Build history of the part. All positions in model axes, mm. A direction names the side the tool comes from. Round coordinates to 2 decimals unless told otherwise and drop trailing zeros. Order: outer loops, then holes, each group sorted by start corner. A loop starts at its lowest first (then second) coordinate and runs counter-clockwise, first axis right, second up. Notation, with made-up numbers: M -16.5,88.25 L 17.5,88.25 A6 ccw 17.5,94.25 Z; hole C 24.5,-25 d2. An arc over 180 degrees is marked long. One line per item, written item: value. Start each with the question number.
Item 1: Band-saw the part on D-D, the plane x = 37. Write the cut outline in (y, z).
Item 2: Pin check, flat tips, straight feed: pin 1 (0.6 mm diameter, centred on x = 26, y = 1, fed in from +Z); pin 2 (3.5 mm diameter, centred on x = 45.48, z = -41.7, fed in from +Y). Stop position of each tip, or through.
Item 3: Tool access for faces 5 (the flat face through (10, 1, -39.701)), 6 (the flat face through (37, 2, -37)), 7 (the flat face through (23, 1, -36.692)): list every direction of +Z, -Z, +X, -X, +Y, -Y with a clear straight run to the whole face (end or side of a thin tool).
Item 4: Probe L1, parallel to Z at x = 11, y = 1.3; L2, parallel to X at y = 0.8, z = -6; L3, parallel to Z at x = 45.48, y = 1.65. List the from-to ranges inside material, lowest first.
Item 5: Two-plate mould, pull along Z, no slides. Class faces 1 (the flat face through (0, 1, -43)), 2 (the flat face through (41.967, 0.986, 18.527)), 3 (the flat face through (10, 1, -43.701)), 4 (the flat face through (4.55, 1, -42)): +Z half, -Z half, draft (parallel to the pull), parting line (faces both ways), or undercut.
Item 6: Band-saw the part on A-A, the plane x = 8.5. Write the cut outline in (y, z).
Item 7: Band-saw the part on C-C, the plane z = -21. Write the cut outline in (x, y).
Item 8: Band-saw the part on B-B, the plane y = 0.6. Write the cut outline in (x, z), then the cut area to 3 significant figures.
```python
from build123d import *

# Parameters (mm, degrees)
SKETCH1_R           = 2
BOSS_EXTRUDE2_DEPTH = 2
CUT_EXTRUDE2_DEPTH  = 9
CUT_EXTRUDE3_DEPTH  = 9


with BuildPart() as part:
    # Sketch1 → Boss-Extrude2 (new body)
    with BuildSketch(Plane(origin=(0, 0, 0), x_dir=(1, 0, 0), z_dir=(0, 1, 0))):
        with BuildLine():
            Line((0, 48.412862342), (0, 37.692030173))
            ThreePointArc((0, 37.692030173), (0.292893219, 36.984923392), (1, 36.692030173))
            Line((1, 36.692030173), (31.48, 36.692030173))
            Line((31.48, 36.692030173), (43.036527631, 36.692030173))
            Line((43.036527631, 36.692030173), (43.036527631, -13.307969827))
            Line((43.036527631, -13.307969827), (38.310297741, -17.310739702))
            Line((38.310297741, -17.310739702), (34.253582629, -17.310739702))
            Line((34.253582629, -17.310739702), (36, -19.267392345))
            Line((36, -19.267392345), (30.071702425, -24.288225334))
            Line((30.071702425, -24.288225334), (54.200832168, -12.602889922))
            Line((54.200832168, -12.602889922), (54.200832168, 10.267562985))
            Line((54.200832168, 10.267562985), (54.200832168, 49.412862342))
            Line((54.200832168, 49.412862342), (41.48, 49.412862342))
            Line((41.48, 49.412862342), (1, 49.412862342))
            ThreePointArc((1, 49.412862342), (0.292893219, 49.119969123), (0, 48.412862342))
        make_face()
        with Locations((45.48, 41.700609081)):
            Circle(SKETCH1_R, mode=Mode.SUBTRACT)
        with BuildLine():
            Line((15, 43.700609081), (4.549516448, 43.700609081))
            Line((4.549516448, 43.700609081), (4.549516448, 39.700609081))
            Line((4.549516448, 39.700609081), (15, 39.700609081))
            ThreePointArc((15, 39.700609081), (17, 41.700609081), (15, 43.700609081))
        make_face(mode=Mode.SUBTRACT)
    extrude(amount=BOSS_EXTRUDE2_DEPTH)

    # Sketch6 → Cut-Extrude2 (cut)
    with BuildSketch(Plane(origin=(0, 2, 0), x_dir=(1, 0, 0), z_dir=(0, 1, 0))):
        Polygon((36, -19.267392345), (38.310297741, -17.310739702), (34.253582629, -17.310739702), align=None)
    extrude(amount=-CUT_EXTRUDE2_DEPTH, mode=Mode.SUBTRACT)

    # Sketch8 → Cut-Extrude3 (cut)
    with BuildSketch(Plane(origin=(0, 2, 0), x_dir=(1, 0, 0), z_dir=(0, 1, 0))):
        Polygon((43.036527631, 36.692030173), (45.036527631, 36.692030173), (45.036527631, -11.115496155), (45.036527631, -11.614116599), (43.036527631, -13.307969827), align=None)
    extrude(amount=-CUT_EXTRUDE3_DEPTH, mode=Mode.SUBTRACT)


solid = part.part
```
Output:
1. outline: M 0,-49.41 L 2,-49.41 L 2,-36.69 L 0,-36.69 Z; M 0,18.42 L 2,18.42 L 2,20.93 L 0,20.93 Z
2. pin 1: stops at z = -36.69
2. pin 2: passes through
3. face 5: +Y, -Y
3. face 6: +Z, -Z, +X, -X, +Y
3. face 7: -X, +Y, -Y
4. L1: z = -49.41 to -43.7, -39.7 to -36.69
4. L2: x = 45.04 to 54.2
4. L3: z = -49.41 to -43.7, -39.7 to 16.83
5. face 1: draft
5. face 2: +Z half
5. face 3: undercut
5. face 4: undercut
6. outline: M 0,-49.41 L 2,-49.41 L 2,-43.7 L 0,-43.7 Z; M 0,-39.7 L 2,-39.7 L 2,-36.69 L 0,-36.69 Z
7. outline: M 45.04,0 L 54.2,0 L 54.2,2 L 45.04,2 Z
8. outline: M 0,-48.41 A1 ccw 1,-49.41 L 54.2,-49.41 L 54.2,12.6 L 30.07,24.29 L 45.04,11.61 L 45.04,-36.69 L 1,-36.69 A1 ccw 0,-37.69 Z; hole M 4.55,-43.7 L 15,-43.7 A2 ccw 15,-39.7 L 4.55,-39.7 Z; hole C 45.48,-41.7 d4
8. area: 1,140 mm²
